Design review of the part built by this model. Coordinates are the model's own, in mm. Face numbers are marked on the shaded views. Give positions to 0.01 mm unless a question says otherwise; leave off trailing zeros. Loops run counter-clockwise (first coordinate to the right, second up) from the corner with the lowest first, then second, coordinate; pieces in that order, holes last. Notation, with made-up numbers: M -2,48 L 25,48 A8 cw 25,55 Z; hole C 12.5,32 d10. An arc over 180 degrees is marked long. Use a Markdown table: item, result. Add a question column.
(1) Draft analysis for pull direction X (two halves, no side actions). For the marked faces 1, 2, 3 and 4, state which applies: pulls with the +X half, pulls with the -X half, needs draft (parallel to the pull), parting line crosses it, or undercut.
(2) Add section C-C, the plane x = 60.5. Give the boundary of the cut face in (y, z).
(3) For probe 1 along X at (y, z) = (7, -30); probe 2 along X at (y, z) = (14.5, -20); probe 3 along Y at (x, z) = (32, -95), list the stretches that pass through material, from the lowest coordinate up.
(4) Add section A-A, the plane z = -9. Give the boundary of the cut face in (x, y) (3 decimals).
(5) Add section B-B, the plane y = 28. Give the boundary of the cut face in (x, z), then the cut area to 3 significant figures.
(6) Insertion check: pin 1 Ø8 at (x, y) = (81, 17.5) entering from +Z; pin 2 Ø10 at (x, z) = (77.5, -86) entering from +Y; pin 3 Ø12 at (y, z) = (22.5, -83) entering from -X. Each pin has a flat end and moves straight along its axis. Give the tip position at first contact, or say it passes through.
(7) Add section D-D, the plane z = -24.5. Give the boundary of the cut face in (x, y).
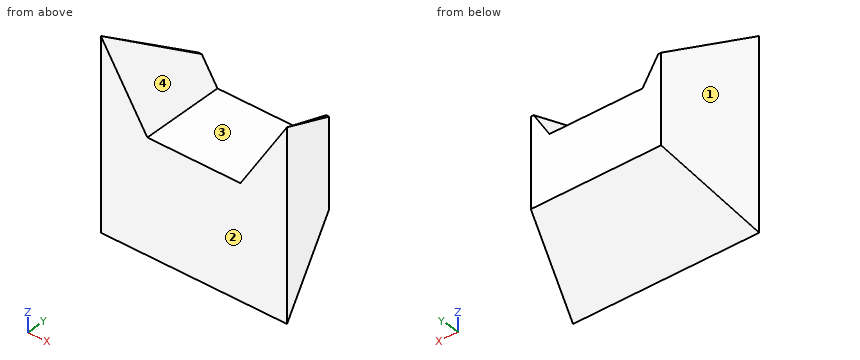
```python
from build123d import *

# Parameters (mm, degrees)
GRUNDK_RPER_DEPTH               = 100
SCHRAEGEN_VORNE_DEPTH           = 100
SCHNITT_LINEAR_AUSTRAGEN4_DEPTH = 45


with BuildPart() as part:
    # Skizze1 → Grundkörper (new body)
    with BuildSketch(Plane.XY):
        Polygon((0, 0), (100, 0), (85, 45), (15, 45), align=None)
    extrude(amount=-GRUNDK_RPER_DEPTH)

    # Skizze2 → Schraegen_vorne (cut)
    with BuildSketch(Plane(origin=(0, 0, 0), x_dir=(0, 0, -1), z_dir=(1, 0, 0))):
        Polygon((100, 0), (73.544212344, 45), (100, 45), align=None)
    schraegen_vorne = extrude(amount=SCHRAEGEN_VORNE_DEPTH, mode=Mode.SUBTRACT)

    # Spiegel_Schraege_hinten: Schraegen_vorne across plane
    add(schraegen_vorne.mirror(Plane.XY.offset(-50)), mode=Mode.SUBTRACT)

    # Skizze4 → Schnitt-Linear austragen4 (cut)
    with BuildSketch(Plane.XZ):
        Polygon((100, 0), (75, -40), (25, -40), (0, 0), align=None)
    extrude(amount=-SCHNITT_LINEAR_AUSTRAGEN4_DEPTH, mode=Mode.SUBTRACT)


solid = part.part
```
Established:
| question | item | result |
|---|---|---|
| 1 | face 1 | pulls with the -X half |
| 1 | face 2 | needs draft |
| 1 | face 3 | undercut |
| 1 | face 4 | undercut |
| 2 | outline | M 0,-100 L 45,-73.54 L 45,-40 L 0,-40 Z |
| 3 | probe 1 | 2.33 to 18.75, 81.25 to 97.67 |
| 3 | probe 2 | 4.83 to 12.5, 87.5 to 95.17 |
| 3 | probe 3 | 0 to 8.5 |
| 4 | outline | M 0,0 L 5.625,0 L 5.625,15.309 L 5.103,15.309 Z; M 94.375,0 L 100,0 L 94.897,15.309 L 94.375,15.309 Z |
| 5 | outline | M 9.33,-83.54 L 90.67,-83.54 L 90.67,-16.46 L 89.71,-16.46 L 75,-40 L 25,-40 L 10.29,-16.46 L 9.33,-16.46 Z |
| 5 | area | 3,930 mm^2 |
| 6 | pin 1 | z = -24 |
| 6 | pin 2 | y = 32.32 |
| 6 | pin 3 | x = 5.5 |
| 7 | outline | M 0,0 L 15.31,0 L 15.31,41.67 L 13.89,41.67 Z; M 84.69,0 L 100,0 L 86.11,41.67 L 84.69,41.67 Z |
